from build123d import *

# Parameters (mm, degrees)
SKETCH1_W                = 30.1752
SKETCH1_H                = 12.7
BOSS_EXTRUDE1_DEPTH      = 6.35
BOSS_EXTRUDE1_DEPTH_BACK = 6.35
SKETCH2_W                = 17.4752
SKETCH2_H                = 6.6675
CUT_EXTRUDE1_DEPTH       = 6.35
CUT_EXTRUDE1_DEPTH_BACK  = 6.35
HOLE1_D                  = 5.36702
HOLE1_DEPTH              = 11.176
HOLE1_CSINK_D            = 6.35
HOLE1_CSINK_ANGLE        = 90
SKETCH5_W                = 2.7051
SKETCH5_H                = 1.524


with BuildPart() as part:
    # Sketch1 → Boss-Extrude1 (new body, two sides)
    with BuildSketch(Plane.XY) as boss_extrude1_sk:
        with Locations((8.7376, 0)):
            Rectangle(SKETCH1_W, SKETCH1_H)
    extrude(amount=BOSS_EXTRUDE1_DEPTH)
    extrude(boss_extrude1_sk.sketch, amount=-BOSS_EXTRUDE1_DEPTH_BACK)

    # Sketch2 → Cut-Extrude1 (cut, two sides)
    with BuildSketch(Plane(origin=(0, 0, 0), x_dir=(1, 0, 0), z_dir=(0, 1, 0))) as cut_extrude1_sk:
        with Locations((2.3876, 0)):
            Rectangle(SKETCH2_W, SKETCH2_H)
    extrude(amount=CUT_EXTRUDE1_DEPTH, mode=Mode.SUBTRACT)
    extrude(cut_extrude1_sk.sketch, amount=-CUT_EXTRUDE1_DEPTH_BACK, mode=Mode.SUBTRACT)

    # Hole1
    with Locations(Plane(origin=(23.8252, 0, 0), x_dir=(0, 0, -1), z_dir=(1, 0, 0))):
        with Locations((0, 0)):
            CounterSinkHole(HOLE1_D / 2, HOLE1_CSINK_D / 2, depth=HOLE1_DEPTH, counter_sink_angle=HOLE1_CSINK_ANGLE)

    # Sketch5 → Hole2 (revolve, cut)
    with BuildSketch(Plane(origin=(12.6492, 0, 0), x_dir=(0, 0, -1), z_dir=(0, 1, 0))):
        with Locations((1.35255, 0.762)):
            Rectangle(SKETCH5_W, SKETCH5_H)
    revolve(axis=Axis((-97.3508, 0, 0), (1, 0, 0)), mode=Mode.SUBTRACT)

    # Sketch7 → Cut-Revolve1 (revolve, cut)
    with BuildSketch(Plane(origin=(0, 0, 0), x_dir=(0, 0, -1), z_dir=(1, 0, 0))):
        Polygon((-6.35, 0), (-6.35, 4.33705), (-5.207, 3.19405), (5.207, 3.19405), (6.35, 4.33705), (6.35, 0), align=None)
    revolve(axis=Axis((0, 0, -6.35), (0, 0, 1)), mode=Mode.SUBTRACT)

    # Sketch8 → Cut-Revolve2 (revolve, cut)
    with BuildSketch(Plane.XY):
        with BuildLine():
            Line((23.8252, 0), (23.8252, 6.35))
            ThreePointArc((23.8252, 6.35), (22.869586956, 9.650754782), (21.2852, 12.7))
            Line((21.2852, 12.7), (30.1752, 12.7))
            Line((30.1752, 12.7), (30.1752, 0))
            Line((30.1752, 0), (23.8252, 0))
        make_face()
    revolve(axis=Axis((30.1752, 0, 0), (-1, 0, 0)), mode=Mode.SUBTRACT)

    # Sketch9 → Cut-Revolve3 (revolve, cut)
    with BuildSketch(Plane.XY):
        with BuildLine():
            Line((-12.7, 0), (-12.7, 12.7))
            Line((-12.7, 12.7), (-3.81, 12.7))
            ThreePointArc((-3.81, 12.7), (-5.394386956, 9.650754782), (-6.35, 6.35))
            Line((-6.35, 6.35), (-6.35, 0))
            Line((-6.35, 0), (-12.7, 0))
        make_face()
    revolve(axis=Axis((-6.35, 0, 0), (-1, 0, 0)), mode=Mode.SUBTRACT)


solid = part.part
Model file for the job. Use its own axes, mm. A direction names the side the tool comes from. Coordinates: 2 decimals unless noted, no trailing zeros. Loops run counter-clockwise (first coordinate to the right, second up) from the corner with the lowest first, then second, coordinate; pieces in that order, holes last. Notation, with made-up numbers: (-38, -25.5) -> (-5, -25.5) arc R33 ccw to (-5, 8.5) -> close; hole circle Ø9 at (54, 88.25). An arc over 180 degrees is marked (long way). Use one line per item in the form item = value. Start each with the question number.
(1) Cut at A-A on x = 0. Give the cut face in (y, z).
(2) Flat gauge pin, fed straight in: pin 1 (4.5 mm diameter, centred on y = 1, z = -1, fed in from -X). Where does the tip first touch, or does it go through?
(3) Cut at B-B on x = 5.5. Give the cut face in (y, z).
(4) Cut at D-D on y = -0.5. Give the number of separate pieces and of enclosed holes in the cut face, and give its area (3 significant figures).
(5) Probe probe 1 along Y at (x, z) = (20.75, 0); probe 2 along Y at (x, z) = (0, -4.45); probe 3 along Z at (x, y) = (3, -4.75). List the from-to ranges inside material, lowest first. Write a range as from..to.
(6) Tool access for faces 4 (the flat face through (12, 6.35, 0)), 5 (the flat face through (4, 0, 3.334)), 6 (the cylindrical face through (11.88, 0.81, -2.58)): list every direction of +Z, -Z, +X, -X, +Y, -Y with a clear straight run to the whole face (end or side of a thin tool).
(7) Pull direction Z, two halves, no side cores. Call faces 1 (the flat face through (12, -6.35, 0)), 2 (the flat face through (4, 0, -3.334)), 3 (the flat face through (9, 0, 6.35)): pulls with the +Z half, pulls with the -Z half, needs draft (parallel to the pull), parting line crosses it, or undercut.
(8) Cut at C-C on x = 20.5. Give the cut face in (y, z).
Values:
q1.outline = (-6.35, -6.35) -> (-4.34, -6.35) -> (-3.19, -5.21) -> (-3.19, -3.33) -> (-6.35, -3.33) -> close; (-6.35, 3.33) -> (-3.19, 3.33) -> (-3.19, 5.21) -> (-4.34, 6.35) -> (-6.35, 6.35) -> close; (3.19, -5.21) -> (4.34, -6.35) -> (6.35, -6.35) -> (6.35, -3.33) -> (3.19, -3.33) -> close; (3.19, 3.33) -> (6.35, 3.33) -> (6.35, 6.35) -> (4.34, 6.35) -> (3.19, 5.21) -> close
q2.pin_1 = 11.13
q3.outline = (-6.35, -6.35) -> (6.35, -6.35) -> (6.35, -3.33) -> (-6.35, -3.33) -> close; (-6.35, 3.33) -> (6.35, 3.33) -> (6.35, 6.35) -> (-6.35, 6.35) -> close
q4.separate_pieces = 4
q4.enclosed_holes = 0
q4.area = 159 mm2
q5.probe_1 = -6.35..-2.68, 2.68..6.35
q5.probe_2 = -6.35..-3.19, 3.19..6.35
q5.probe_3 = -6.35..-3.33, 3.33..6.35
q6.face_4 = +Z, -Z, +X, -X, +Y
q6.face_5 = -X, +Y, -Y
q6.face_6 = -X
q7.face_1 = needs draft
q7.face_2 = undercut
q7.face_3 = pulls with the +Z half
q8.outline = (-6.35, -6.35) -> (6.35, -6.35) -> (6.35, 6.35) -> (-6.35, 6.35) -> close; hole circle Ø5.37 at (0, 0)
